The model under review builds one solid part; all positions refer to its coordinate system, in mm. A direction names the side the tool comes from. Coordinates: 2 decimals unless noted, no trailing zeros. Write each loop counter-clockwise with the first axis right and the second up, starting at its lowest first coordinate (ties: lowest second). Pieces come first, ordered by that corner, then holes.
1) Machinability: for faces 5 (the flat face through (23, 0, -14.05)), 6 (the flat face through (20.25, 0, 13)), 7 (the flat face through (23, -3.25, -16)), 8 (the flat face through (13, -1, 19.55)), which of the approach directions +Z, -Z, +X, -X, +Y, -Y give a long, thin tool a straight path to every point of the face, cutting with its end or side? Answer none if there is none.
2) For P1, Ø6, axis at y = -6.5, z = 0.5, coming from the +X side; P2, Ø6, axis at x = 25, y = 0.5, coming from the +Z side; P3, Ø3, axis at y = -3.5, z = 12, coming from the -X side; P4, Ø2.5, axis at x = 25.25, y = 5, coming from the +Z side, all flat-tipped, find the tip position at first contact; note any pin that passes through.
3) Add section A-A, the plane x = 25.25. State the section outline as (y, z) points, then the cut area to 3 significant figures.
4) Mouldability with a two-part tool opening along X and no side actions: class faces 1 (the flat face through (23, 3, -16)), 2 (the cylindrical face through (27.396, -5.676, 7.318)), 3 (the cylindrical face through (6.853, 0.132, 21.719)), 4 (the cylindrical face through (-23.104, -5.676, 7.318)) as released by +X, released by -X, zero draft, split by the parting line, or undercut.
5) Add section B-B, the plane x = -25.25. State the section outline as (y, z) points.
6) For line 1 (X direction, y = 5, z = 8.05); line 2 (Y direction, x = 25.25, z = 7.5); line 3 (Z direction, x = 23, y = -7), list the stretches that pass through material, from the lowest coordinate up.
7) Add section C-C, the plane z = -8.05. State the section outline as (x, y) points, then the cut area to 3 significant figures.
8) Add section D-D, the plane z = 7. State the section outline as (x, y) points.
from build123d import *

# Parameters (mm, degrees)
F0_W      = 40.5
F0_H      = 36.1
F1_DEPTH  = 10
F3_W      = 7.5
F3_H      = 20
F3_R      = 2.25
F4_DEPTH  = 2.5
F5_R      = 7.25
F6_DEPTH  = 1.5
F6_TAPER  = 33
F8_R      = 3
F9_DEPTH  = 4.4
F10_R     = 2.5
F11_DEPTH = 2
F12_W     = 6.25
F12_H     = 4
F13_DEPTH = 6


# Not quite as in the source:
# - a feature names something its author has since deleted; it is built from what else it names


with BuildPart() as f1:
    # F0 (on Front) → F1 (new body, symmetric)
    with BuildSketch(Plane.XZ):
        Rectangle(F0_W, F0_H)
    extrude(amount=F1_DEPTH, both=True)

    # F3 (on offset) → F4 (join)
    with BuildSketch(Plane(origin=(0, 0, 8.55), x_dir=(1, 0, 0), z_dir=(0, 0, -1))):
        with Locations((-24, 0)):
            Rectangle(F3_W, F3_H)
        with Locations((-25.25, -5)):
            Circle(F3_R, mode=Mode.SUBTRACT)
        with Locations((-25.25, 5)):
            Circle(F3_R, mode=Mode.SUBTRACT)
        with Locations((24, 0)):
            Rectangle(F3_W, F3_H)
        with Locations((25.25, -5)):
            Circle(F3_R, mode=Mode.SUBTRACT)
        with Locations((25.25, 5)):
            Circle(F3_R, mode=Mode.SUBTRACT)
    extrude(amount=F4_DEPTH)

    # F5 (on face) → F6 (join)
    with BuildSketch(Plane.XY.offset(18.05)):
        with Locations((9.85, 0)):
            Circle(F5_R)
    extrude(amount=F6_DEPTH, taper=F6_TAPER)

    # F8 (on face) → F9 (join, through all)
    with BuildSketch(Plane.XY.offset(19.55)):
        with Locations((9.85, 0)):
            Circle(F8_R)
    extrude(amount=F9_DEPTH)

    # F10 (on face) → F11 (cut)
    with BuildSketch(Plane.YZ.offset(20.25)):
        with Locations((0, -8.05)):
            Circle(F10_R)
    extrude(amount=-F11_DEPTH, mode=Mode.SUBTRACT)

    # F12 (on face) → F13 (join)
    with BuildSketch(Plane.YZ.offset(20.25)):
        with Locations((-0.125, -16.05)):
            Rectangle(F12_W, F12_H)
    extrude(amount=F13_DEPTH)


solid = f1.part
Geometry results:
1. face 5: +X, +Y, -Y
1. face 6: +Z, +X, +Y, -Y
1. face 7: -Z, +X, -Y
1. face 8: +Z
2. P1: stops at x = 20.25
2. P2: stops at z = 8.55
2. P3: stops at x = -20.25
2. P4: passes through
3. outline: (-10, 6.05) - (-7.25, 6.05) - (-7.25, 8.55) - (-10, 8.55) - close; (-3.25, -18.05) - (3, -18.05) - (3, -14.05) - (-3.25, -14.05) - close; (-2.75, 6.05) - (2.75, 6.05) - (2.75, 8.55) - (-2.75, 8.55) - close; (7.25, 6.05) - (10, 6.05) - (10, 8.55) - (7.25, 8.55) - close
3. area: 52.5 mm2
4. face 1: zero draft
4. face 2: undercut
4. face 3: split by the parting line
4. face 4: undercut
5. outline: (-10, 6.05) - (-7.25, 6.05) - (-7.25, 8.55) - (-10, 8.55) - close; (-2.75, 6.05) - (2.75, 6.05) - (2.75, 8.55) - (-2.75, 8.55) - close; (7.25, 6.05) - (10, 6.05) - (10, 8.55) - (7.25, 8.55) - close
6. line 1: x = -27.75 to -27.5, -23 to 23, 27.5 to 27.75
6. line 2: y = -10 to -7.25, -2.75 to 2.75, 7.25 to 10
6. line 3: z = 6.05 to 8.55
7. outline: (-20.25, -10) - (20.25, -10) - (20.25, -2.5) - (18.25, -2.5) - (18.25, 2.5) - (20.25, 2.5) - (20.25, 10) - (-20.25, 10) - close
7. area: 800 mm2
8. outline: (-27.75, -10) - (27.75, -10) - (27.75, 10) - (-27.75, 10) - close; hole circle Ø4.5 at (-25.25, -5); hole circle Ø4.5 at (-25.25, 5); hole circle Ø4.5 at (25.25, -5); hole circle Ø4.5 at (25.25, 5)
